Design review of the part built by this model. Coordinates are the model's own, in mm. Face numbers are marked on the shaded views. A direction names the side the tool comes from. Coordinates: 2 decimals unless noted, no trailing zeros. Write each loop counter-clockwise with the first axis right and the second up, starting at its lowest first coordinate (ties: lowest second). Pieces come first, ordered by that corner, then holes. Notation, with made-up numbers: M -9.75,44.25 L 47.25,44.25 A22 cw 47.25,70.25 Z; hole C 5.5,52 d7. An arc over 180 degrees is marked long. One line per question, with ' | ' between items.
from build123d import *

# Parameters (mm, degrees)
F0_W     = 203.2
F0_H     = 127
F1_DEPTH = 127
F3_DEPTH = 76.2
F4_SIZE2 = 101.6
F4_SIZE  = 76.2
F5_R     = 5.08
F6_R     = 15.24
F7_DEPTH = 50.8
F8_R     = 15.24
F9_DEPTH = 127


with BuildPart() as f1:
    # F0 (on Front) → F1 (new body)
    with BuildSketch(Plane.XZ):
        with Locations((41.3226257026, 20.5530026861)):
            Rectangle(F0_W, F0_H)
    extrude(amount=F1_DEPTH)

    # F2 (on face) → F3 (cut)
    with BuildSketch(Plane.XZ.offset(127)):
        Polygon((142.9226257026, 84.0530026861), (34.8217822611, 84.0530026861), (34.8217822611, 38.4303182364), (0, 38.4303182364), (0, -42.9469973139), (142.9226257026, -42.9469973139), align=None)
    extrude(amount=-F3_DEPTH, mode=Mode.SUBTRACT)

    # F4
    f4_edges = [f1.edges().sort_by_distance(p)[0] for p in [
        (142.922626, -25.4, 84.053003),
    ]]
    f4_side = f1.faces().sort_by_distance((19.028994, -51.591204, 84.053003))[0]
    chamfer(f4_edges, length=F4_SIZE, length2=F4_SIZE2, reference=f4_side)

    # F5
    f5_edges = [f1.edges().sort_by_distance(p)[0] for p in [
        (34.821782, -88.9, 84.053003),
        (0, -127, -2.25834),
        (50.772204, -50.8, 84.053003),
        (34.821782, -50.8, 61.24166),
        (34.821782, -127, 61.24166),
        (17.410891, -127, 38.430318),
        (-30.138687, -127, -42.946997),
        (-60.277374, -127, 20.553003),
        (-12.727796, -127, 84.053003),
        (3.222626, 0, 84.053003),
        (66.722626, -25.4, 84.053003),
        (-60.277374, -63.5, 84.053003),
        (0, -50.8, -2.25834),
        (0, -88.9, 38.430318),
        (0, -88.9, -42.946997),
        (142.922626, 0, -30.246997),
        (142.922626, -25.4, -17.546997),
        (142.922626, -25.4, -42.946997),
        (142.922626, -50.8, -30.246997),
        (41.322626, 0, -42.946997),
        (-60.277374, 0, 20.553003),
        (-60.277374, -63.5, -42.946997),
        (34.821782, -88.9, 38.430318),
        (17.410891, -50.8, 38.430318),
        (71.461313, -50.8, -42.946997),
    ]]
    fillet(f5_edges, radius=F5_R)

    # F6 (on face) → F7 (cut, through all)
    with BuildSketch(Plane.XZ.offset(50.8)):
        with Locations((55.88, 2.7730026861)):
            Circle(F6_R)
    extrude(amount=-F7_DEPTH, mode=Mode.SUBTRACT)

    # F8 (on face) → F9 (cut, through all)
    with BuildSketch(Plane.XY.offset(84.0530026861)):
        with Locations((-18.4064079076, -68.5097798705)):
            Circle(F8_R)
    extrude(amount=-F9_DEPTH, mode=Mode.SUBTRACT)


solid = f1.part
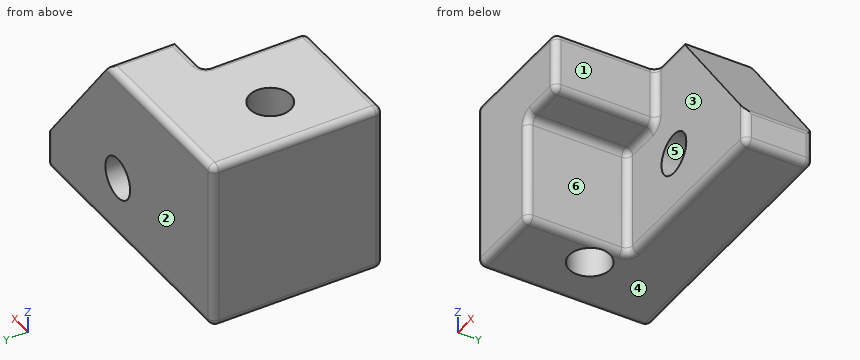
1. Draft analysis for pull direction Z (two halves, no side actions). For the marked faces 4, 5 and 6, state which applies: pulls with the +Z half, pulls with the -Z half, needs draft (parallel to the pull), parting line crosses it, or undercut.
Answer sheet:
face 4: pulls with the -Z half | face 5: undercut | face 6: needs draft
2. Take a section at D-D (y = -116.5). Write out the cut boundary in (x, z), then the cut area to 3 significant figures.
Answer sheet:
outline: M -60.28,-37.87 A5.08 ccw -55.2,-42.95 L -5.08,-42.95 A5.08 ccw 0,-37.87 L 0,33.35 A5.08 cw 5.08,38.43 L 29.74,38.43 A5.08 ccw 34.82,43.51 L 34.82,78.97 A5.08 ccw 29.74,84.05 L -55.2,84.05 A5.08 ccw -60.28,78.97 Z | area: 9,220 mm^2
3. Take a section at C-C (y = -81.5). Write out the cut boundary in (x, z), then the cut area to 3 significant figures.
Answer sheet:
outline: M -60.28,-37.87 A5.08 ccw -55.2,-42.95 L -26.38,-42.95 L -26.38,84.05 L -55.2,84.05 A5.08 ccw -60.28,78.97 Z; M -10.44,-42.95 L -5.08,-42.95 A5.08 ccw 0,-37.87 L 0,33.35 A5.08 cw 5.08,38.43 L 29.74,38.43 A5.08 ccw 34.82,43.51 L 34.82,78.97 A5.08 ccw 29.74,84.05 L -10.44,84.05 Z | area: 7,200 mm^2
4. Take a section at B-B (x = 55.88). Write out the cut boundary in (y, z), then the cut area to 3 significant figures.
Answer sheet:
outline: M -50.8,-37.87 A5.08 ccw -45.72,-42.95 L -5.08,-42.95 A5.08 ccw 0,-37.87 L 0,-12.47 L -50.8,-12.47 Z; M -50.8,18.01 L 0,18.01 L 0,78.97 A5.08 ccw -5.08,84.05 L -45.72,84.05 A5.08 ccw -50.8,78.97 Z | area: 4,880 mm^2
5. Take a section at A-A (z = 6). Write out the cut boundary in (x, y), then the cut area to 3 significant figures.
Answer sheet:
outline: M -60.28,-121.92 A5.08 ccw -55.2,-127 L -5.08,-127 A5.08 ccw 0,-121.92 L 0,-55.88 A5.08 cw 5.08,-50.8 L 40.99,-50.8 L 40.99,0 L -55.2,0 A5.08 ccw -60.28,-5.08 Z; M 70.77,-50.8 L 125.26,-50.8 L 125.26,0 L 70.77,0 Z; hole C -18.41,-68.51 d30.48 | area: 11,800 mm^2
6. Insertion check: pin 1 Ø4 at (x, y) = (97.5, -46) entering from +Z; pin 2 Ø19.5 at (x, y) = (23, -102.5) entering from -Z; pin 3 Ø1 at (x, y) = (99.5, -37) entering from +Z. Each pin has a flat end and moves straight along its axis. Give the tip position at first contact, or say it passes through.
Answer sheet:
pin 1: z = 45.68 | pin 2: z = 38.43 | pin 3: z = 41.02
7. Tool access review of the marked faces 1, 2 and 3: name each direction out of +Z, -Z, +X, -X, +Y, -Y from which nothing blocks a thin tool from reaching the whole face with its end or side.
Answer sheet:
face 1: +Z, -Z, +X, -Y | face 2: +Z, -Z, +X, -X, +Y | face 3: -Z, +X, -Y
8. To check wall thickness, follow line 1 along Z through (x, y) = (55.88, -31); line 2 along Z through (x, y) = (55, -25); line 3 along Y through (x, z) = (88, -32). State the ranges of each line that lie inside material, in increasing order. Write a range as [from, to].
Answer sheet:
line 1: [-42.95, -12.47], [18.01, 84.05] | line 2: [-42.95, -12.44], [17.99, 84.05] | line 3: [-50.8, 0]
